Drawing for the job (mm, zero at the part's lowest x, y, z). A direction names the side the tool comes from. Coordinates: 2 decimals unless noted, no trailing zeros. Loops run counter-clockwise (first coordinate to the right, second up) from the corner with the lowest first, then second, coordinate; pieces in that order, holes last.
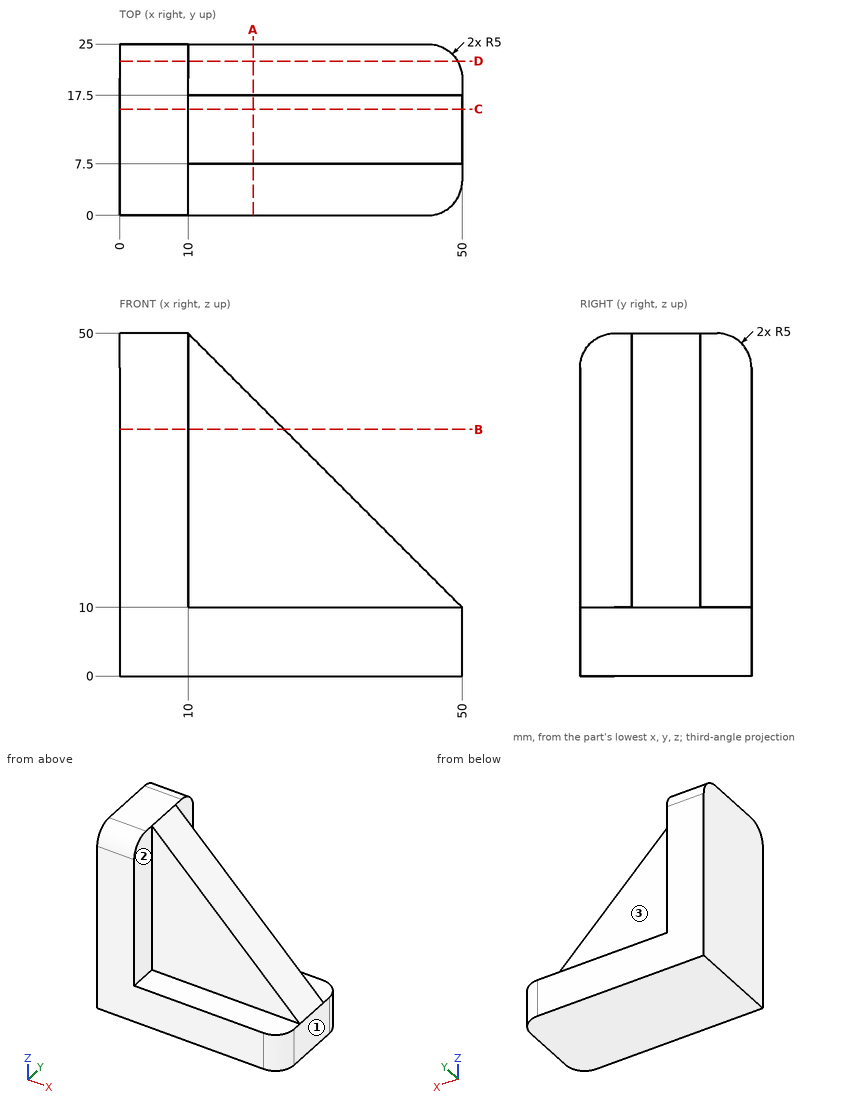
Q1. Probe line 1 (X direction, y = 5.5, z = 25); line 2 (Y direction, x = 16.5, z = 23.5). List the from-to ranges inside material, lowest first.
Q2. Drop flat-ended pins along their axis: P1, Ø5, axis at x = 36.5, y = 17, coming from the +Z side; P2, Ø4, axis at x = 23, z = 38, coming from the -Y side; P3, Ø6, axis at x = 28.5, y = 5, coming from the +Z side. Give the stop position or say it passes through.
Q3. Saw through at D-D (y = 22.5). List the corners of the cut face in (x, z), plus the area to 3 significant figures.
Q4. Saw through at B-B (z = 36). List the corners of the cut face in (x, y), plus the area to 3 significant figures.
Q5. Saw through at A-A (x = 19.5). List the corners of the cut face in (y, z), plus the area to 3 significant figures.
Q6. Saw through at C-C (y = 15.5). List the corners of the cut face in (x, z).
Q7. Tool access for the marked faces 1, 2 and 3: list every direction of +Z, -Z, +X, -X, +Y, -Y with a clear straight run to the whole face (end or side of a thin tool).
Checked values:
1. line 1: x = 0 to 10
1. line 2: y = 7.5 to 17.5
2. P1: stops at z = 26
2. P2: stops at y = 7.5
2. P3: stops at z = 33.16
3. outline: (0, 0) - (49.33, 0) - (49.33, 10) - (10, 10) - (10, 49.33) - (0, 49.33) - close
3. area: 887 mm2
4. outline: (0, 0) - (10, 0) - (10, 7.5) - (24, 7.5) - (24, 17.5) - (10, 17.5) - (10, 25) - (0, 25) - close
4. area: 390 mm2
5. outline: (0, 0) - (25, 0) - (25, 10) - (17.5, 10) - (17.5, 40.5) - (7.5, 40.5) - (7.5, 10) - (0, 10) - close
5. area: 555 mm2
6. outline: (0, 0) - (50, 0) - (50, 10) - (10, 50) - (0, 50) - close
7. face 1: +Z, -Z, +X, +Y, -Y
7. face 2: +Z, +X, -Y
7. face 3: +Z, +X, +Y
